Autodesk Inventor part; units mm, degrees
ref_plane "YZ Plane" through (0, 0, 0) normal (1, 0, 0) x (0, 1, 0)
ref_plane "XZ Plane" through (0, 0, 0) normal (0, 1, 0) x (-1, 0, 0)
ref_plane "XY Plane" through (0, 0, 0) normal (0, 0, 1) x (1, 0, 0)
sketch "Sketch1" plane through (0, 0, 0) normal (0, 1, 0) x (-1, 0, 0)
  line L0 (-6.6677, 20.126) -> (13.7323, 20.126)
  line L1 (13.7323, 20.126) -> (13.7323, -25.074)
  line L2 (13.7323, -25.074) -> (-6.6677, -25.074)
  line L3 (-6.6677, -25.074) -> (-6.6677, 20.126)
  line L4 (15.2323, -26.574) -> (15.2323, 21.626)
  line L5 (15.2323, 21.626) -> (-8.1677, 21.626)
  line L6 (-8.1677, 21.626) -> (-8.1677, -26.574)
  line L7 (-8.1677, -26.574) -> (15.2323, -26.574)
  point P0 (0, 0)
  dimension "d0" = 45.2
  dimension "d1" = 20.4
  dimension "d2" = 1.5
extrude "Extrusion1" add sketch "Sketch1" along normal blind 20
sketch "Sketch2" plane through (8.1677, 0, 21.626) normal (1, 0, 0) x (0, 0, -1)
  line L0 (19.1022, 10.5) -> (29.1022, 10.5)
  line L1 (29.1022, 10.5) -> (29.1022, 5.5)
  line L2 (29.1022, 5.5) -> (19.1022, 5.5)
  line L3 (19.1022, 5.5) -> (19.1022, 10.5)
  line L4 (30.6022, 12) -> (17.6022, 12)
  line L5 (17.6022, 12) -> (17.6022, 4)
  line L6 (17.6022, 4) -> (30.6022, 4)
  line L7 (30.6022, 4) -> (30.6022, 12)
  line L8 (0, 0) -> (0, 20)
  line L9 (48.2, 0) -> (48.2, 20)
  line L10 (0, 20) -> (48.2, 20)
  point P0 (21.626, 0)
  dimension "d5" = 10
  dimension "d6" = 5
  dimension "d7" = 1.5
  dimension "d8" = 17.6022
  dimension "d9" = 17.5978
  dimension "d10" = 8
extrude "Extrusion2" cut sketch "Sketch2" against normal blind 6 contours L0 L1 L2 L3 | L7 L6 L5 L4
extrude "Extrusion3" add sketch "Sketch1" along normal blind 4 contours L0 L1 L2 L3
sketch "Sketch3" plane through (0, 20, 0) normal (0, 1, 0) x (1, 0, 0)
  line L0 (-13.7323, -20.126) -> (-13.7323, 25.074)
  line L1 (-15.2323, 26.574) -> (-15.2323, -21.626)
  line L2 (-13.7323, -20.126) -> (-15.2323, -20.126)
  line L3 (-15.2323, -20.126) -> (-15.2323, 25.074)
  line L4 (-15.2323, 25.074) -> (-13.7323, 25.074)
  line L5 (-13.7323, 25.074) -> (-13.7323, -20.126)
  point P0 (0, 0)
  dimension "d17" = 0
extrude "Extrusion4" cut sketch "Sketch3" against normal blind 16
sketch "Sketch4" plane through (0, 20, 0) normal (0, 1, 0) x (1, 0, 0)
  line L0 (-15.2323, -20.126) -> (-15.2323, -21.626)
  line L1 (-15.2323, -21.626) -> (8.1677, -21.626)
  line L2 (-15.2323, -20.126) -> (-10.2323, -20.126)
  line L3 (-10.2323, -20.126) -> (-10.2323, -21.626)
  line L4 (-10.2323, -21.626) -> (-15.2323, -21.626)
  line L5 (-15.2323, -21.626) -> (-15.2323, -20.126)
  line L6 (6.6677, -20.126) -> (-15.2323, -20.126)
  line L7 (8.1677, -21.626) -> (3.1677, -21.626)
  line L8 (3.1677, -21.626) -> (3.1677, -20.126)
  line L9 (3.1677, -20.126) -> (8.1677, -20.126)
  line L10 (8.1677, -20.126) -> (8.1677, -21.626)
  line L11 (8.1677, 26.574) -> (-15.2323, 26.574)
  line L12 (-15.2323, 25.074) -> (6.6677, 25.074)
  line L13 (-15.2323, 26.574) -> (-10.2323, 26.574)
  line L14 (-10.2323, 26.574) -> (-10.2323, 25.074)
  line L15 (-10.2323, 25.074) -> (-15.2323, 25.074)
  line L16 (-15.2323, 25.074) -> (-15.2323, 26.574)
  line L17 (8.1677, -21.626) -> (8.1677, 26.574)
  line L18 (8.1677, 26.574) -> (3.1677, 26.574)
  line L19 (3.1677, 26.574) -> (3.1677, 25.074)
  line L20 (3.1677, 25.074) -> (8.1677, 25.074)
  line L21 (8.1677, 25.074) -> (8.1677, 26.574)
  point P0 (0, 0)
  dimension "d18" = 5
  dimension "d19" = 5
  dimension "d20" = 5
  dimension "d21" = 5
extrude "Extrusion5" add sketch "Sketch4" along normal blind 3 contours L2 L3 L1 L0 | L20 L12 L19 L11 L17 | L6 L9 L10 L1 L8 | L14 L12 L16 L11
properties part number "US_Casis"
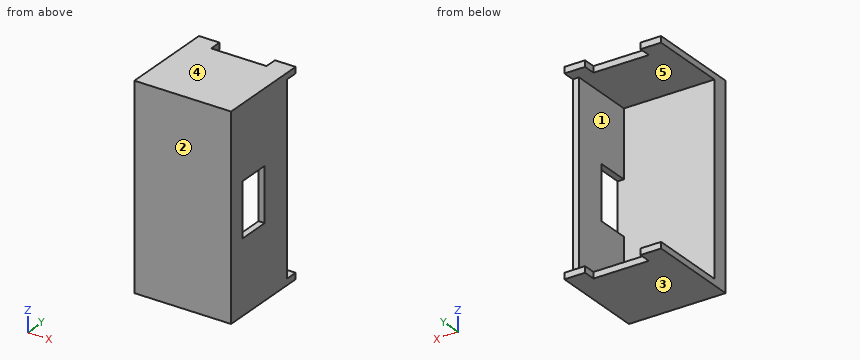
The model under review builds one solid part; all positions refer to its coordinate system, in mm. Face numbers are marked on the shaded views. A direction names the side the tool comes from. Give positions to 0.01 mm unless a question says otherwise; leave off trailing zeros. Write each loop counter-clockwise with the first axis right and the second up, starting at its lowest first coordinate (ties: lowest second). Pieces come first, ordered by that corner, then holes. Notation, with made-up numbers: M 83,62 L 120,62 A26 ccw 120,95 Z; hole C 86,11 d6. An arc over 180 degrees is marked long. Write item = value, one per line. Start each with the question number.
Q1. We need section B-B (z = -3). State the section outline as (x, y) points.
Q2. Clearance check with flat-ended pins moving along their axes: pin 1 (8 mm diameter, centred on y = 11.5, z = 1, fed in from -X); pin 2 (8 mm diameter, centred on x = -12, z = 1.5, fed in from +Y); pin 3 (0.8 mm diameter, centred on x = -1.5, z = -26, fed in from +Y); pin 4 (10 mm diameter, centred on y = 11, z = 0.5, fed in from +X). State where each tip first meets the part, or that it passes through.
Q3. Mouldability with a two-part tool opening along Z and no side actions: class the marked faces 1, 2 and 3 as released by +Z, released by -Z, zero draft, split by the parting line, or undercut.
Q4. We need section C-C (x = 6). State the section outline as (y, z) points.
Q5. We need section A-A (y = 5.25). State the section outline as (x, z) points.
Q6. Machinability: for the marked faces 4 and 5, which of the approach directions +Z, -Z, +X, -X, +Y, -Y give a long, thin tool a straight path to every point of the face, cutting with its end or side? Answer none if there is none.
Q7. For line 1 (Z direction, x = 0.25, y = 12.25); line 2 (Y direction, x = 6.5, z = 15.5); line 3 (X direction, y = 19.75, z = -9), list the stretches that pass through material, from the lowest coordinate up.
Q8. We need section D-D (y = 21). State the section outline as (x, z) points.
Result set:
q1.outline = M -15.23,0 L 8.17,0 L 8.17,4 L -15.23,4 Z; M 6.67,12 L 8.17,12 L 8.17,20 L 6.67,20 Z
q2.pin_1 = 6.67
q2.pin_2 = 4
q2.pin_3 = 20
q2.pin_4 = 8.17
q3.face_1 = undercut
q3.face_2 = zero draft
q3.face_3 = released by -Z
q4.outline = M 0,-26.57 L 23,-26.57 L 23,-25.07 L 4,-25.07 L 4,20.13 L 23,20.13 L 23,21.63 L 0,21.63 Z
q5.outline = M -15.23,-26.57 L 8.17,-26.57 L 8.17,-8.98 L 6.67,-8.98 L 6.67,-25.07 L -15.23,-25.07 Z; M -15.23,20.13 L 6.67,20.13 L 6.67,4.02 L 8.17,4.02 L 8.17,21.63 L -15.23,21.63 Z
q6.face_4 = +Z, +X, -X, +Y, -Y
q6.face_5 = -X, +Y
q7.line_1 = -26.57 to -25.07, 20.13 to 21.63
q7.line_2 = 0 to 4
q7.line_3 = 6.67 to 8.17
q8.outline = M -15.23,-26.57 L -10.23,-26.57 L -10.23,-25.07 L -15.23,-25.07 Z; M -15.23,20.13 L -10.23,20.13 L -10.23,21.63 L -15.23,21.63 Z; M 3.17,-26.57 L 8.17,-26.57 L 8.17,-25.07 L 3.17,-25.07 Z; M 3.17,20.13 L 8.17,20.13 L 8.17,21.63 L 3.17,21.63 Z
